Could you check a few things on this drawing? It's one solid part, dimensions in mm from its lowest x, y, z. A direction names the side the tool comes from. Give positions to 0.01 mm unless a question says otherwise; leave off trailing zeros. Loops run counter-clockwise (first coordinate to the right, second up) from the corner with the lowest first, then second, coordinate; pieces in that order, holes last. Notation, with made-up numbers: (-32.5, 57) - (-2.5, 57) arc R23 cw to (-2.5, 85) - close; hole circle Ø5 at (55.5, -28). An arc over 180 degrees is marked (long way). Answer as a JSON object with one key per item and string values.
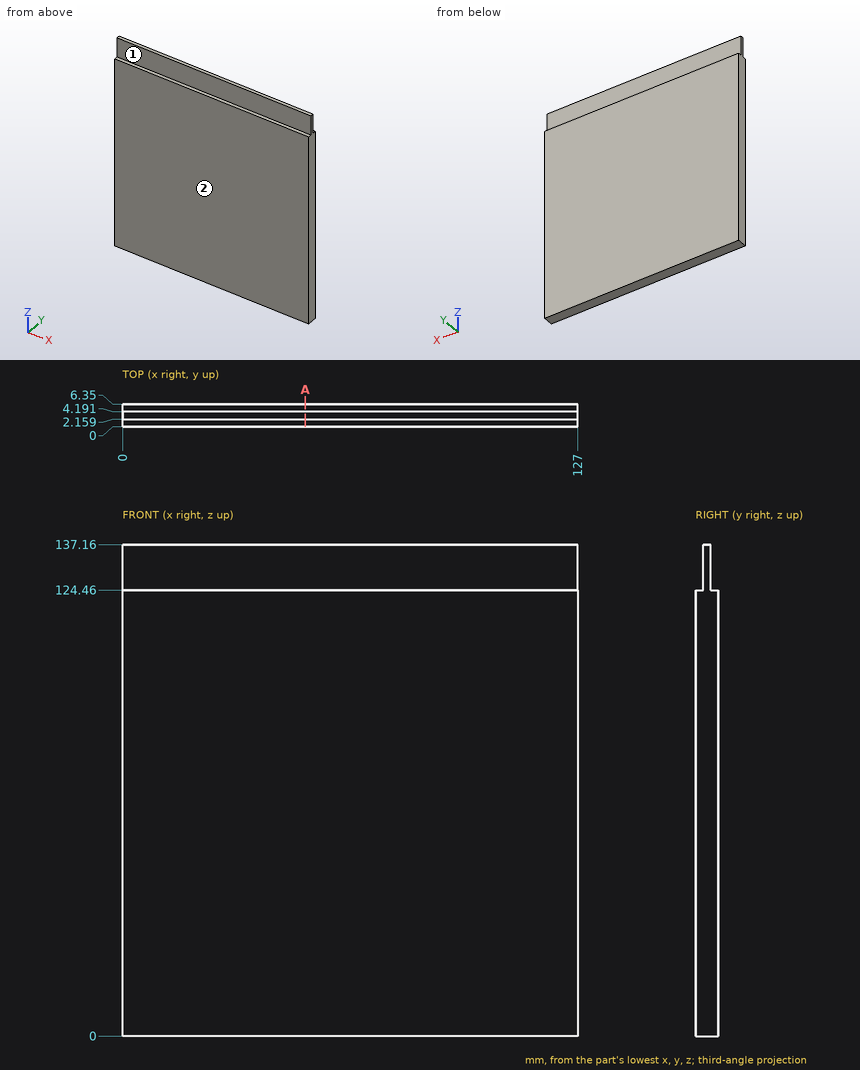
1) I'm going to push flat-ended pins straight in: P1, Ø5, axis at x = 71.5, z = 90, coming from the -Y side; P2, Ø1.7, axis at x = 91, y = 5.5, coming from the +Z side. Where does each tip first touch, or does it pass through?
Check sheet entries:
{"P1": "y = 0", "P2": "z = 124.46"}
2) Imagine slicing it at A-A on x = 51. Write out the boundary of the cut face in (y, z).
Check sheet entries:
{"outline": "(0, 0) - (6.35, 0) - (6.35, 124.46) - (4.19, 124.46) - (4.19, 137.16) - (2.16, 137.16) - (2.16, 124.46) - (0, 124.46) - close"}
3) Which directions (+Z, -Z, +X, -X, +Y, -Y) give clear straight access to the entire face, cutting with the end or side of a thin tool? Please do the marked faces 1 and 2.
Check sheet entries:
{"face 1": "+Z, +X, -X, -Y", "face 2": "+Z, -Z, +X, -X, -Y"}
4) I need wall thicknesses on L1, parallel to Z at x = 73, y = 4.5. Which ranges of the line are inside material? Lowest first, please.
Check sheet entries:
{"L1": "0 to 124.46"}
